from build123d import *

# Parameters (mm, degrees)
BOSS_EXTRUDE3_DEPTH = 10
BOSS_EXTRUDE4_DEPTH = 20
SKETCH2_R           = 2
SKETCH2_R_2         = 3
CUT_EXTRUDE1_DEPTH  = 40
FILLET3_R           = 10
FILLET4_R           = 10
FILLET5_R           = 5
FILLET6_R           = 5
FILLET7_R           = 5
FILLET8_R           = 5


with BuildPart() as part:
    # Sketch1 → Boss-Extrude3 (new, symmetric)
    with BuildSketch(Plane.XY):
        with BuildLine():
            Line((-6.014924663, 62.244051207), (6.208553437, 44.207596014))
            ThreePointArc((6.208553437, 44.207596014), (7.257156315, 41.893061598), (7.472748917, 39.361232736))
            Line((7.472748917, 39.361232736), (2.362176037, -20.425844843))
            ThreePointArc((2.362176037, -20.425844843), (7.015315923, -46.134373754), (24, -65.986342835))
            Line((24, -65.986342835), (31.161941742, -80.882336991))
            ThreePointArc((31.161941742, -80.882336991), (1.523988114, -56.838882139), (-7.619240262, -19.78625212))
            Line((-7.619240262, -19.78625212), (-7.50208553, 38.961677125))
            Line((-7.50208553, 38.961677125), (-13.173612773, 58.905900119))
            ThreePointArc((-13.173612773, 58.905900119), (-11.01662621, 63.625231148), (-6.014924663, 62.244051207))
        make_face()
        with BuildLine():
            Line((-7.499985087, 40.014956421), (-7.500014913, 40))
            ThreePointArc((-7.500014913, 40), (-7.499996272, 40.007478214), (-7.499985087, 40.014956421))
        make_face(mode=Mode.SUBTRACT)
    extrude(amount=BOSS_EXTRUDE3_DEPTH, both=True)

    # Sketch1<4> → Boss-Extrude4 (add, symmetric)
    with BuildSketch(Plane.XY):
        with BuildLine():
            ThreePointArc((25.760539384, -46.570125255), (39.455220381, -67.725242398), (47.426258953, -91.632266743))
            Line((47.426258953, -91.632266743), (38.413830656, -95.965410657))
            Line((38.413830656, -95.965410657), (31.161941742, -80.882336991))
            Line((31.161941742, -80.882336991), (24, -65.986342835))
            Line((24, -65.986342835), (16.748111086, -50.903269169))
            Line((16.748111086, -50.903269169), (25.760539384, -46.570125255))
        make_face()
    extrude(amount=BOSS_EXTRUDE4_DEPTH, both=True)

    # Sketch2 → Cut-Extrude1 (cut)
    with BuildSketch(Plane.XY.offset(10)):
        with Locations((-9.326153163, 60)):
            Circle(SKETCH2_R)
        with Locations((0, 40)):
            Circle(SKETCH2_R_2)
    extrude(amount=-CUT_EXTRUDE1_DEPTH, mode=Mode.SUBTRACT)

    # Fillet3
    fillet3_edges = [part.edges().sort_by_distance(p)[0] for p in [
        (-7.50208553, 38.961677125, 0),
    ]]
    fillet(fillet3_edges, radius=FILLET3_R)

    # Fillet4
    # the kernel refuses this fillet: 10 mm, written as the material it adds along each edge
    with BuildSketch(Plane(origin=(-7.619240262, -19.78625212, -10), x_dir=(0.0019941894265581785, 0.9999980116022886, 0), z_dir=(0, 0, 1))) as fillet4_piece_1:
        with BuildLine():
            CenterArc((0.38347882, 10), FILLET4_R, 265.770794781, 4.229205219)
            ThreePointArc((-0.353986639, 0.027229838), (-0.176973179, 0.013876746), (0, 0))
            Line((0, 0), (0.38347882, 0))
        make_face()
    extrude(amount=20)

    # Fillet5
    fillet5_edges = [part.edges().sort_by_distance(p)[0] for p in [
        (25.760539384, -46.570125255, 0),
    ]]
    fillet(fillet5_edges, radius=FILLET5_R)

    # Fillet6
    fillet6_edges = [part.edges().sort_by_distance(p)[0] for p in [
        (47.426258953, -91.632266743, 0),
    ]]
    fillet(fillet6_edges, radius=FILLET6_R)

    # Fillet7
    fillet7_edges = [part.edges().sort_by_distance(p)[0] for p in [
        (16.748111086, -50.903269169, 0),
    ]]
    fillet(fillet7_edges, radius=FILLET7_R)

    # Fillet8
    fillet8_edges = [part.edges().sort_by_distance(p)[0] for p in [
        (38.413830656, -95.965410657, 0),
    ]]
    fillet(fillet8_edges, radius=FILLET8_R)


solid = part.part
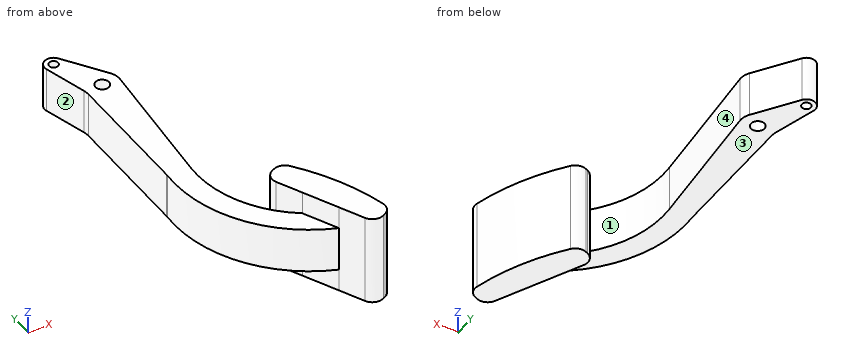
The listing builds one solid part. Answer for the finished solid, in the listing's coordinates (mm). Face numbers are marked on the shaded views. Give positions to 0.01 mm unless a question says otherwise; leave off trailing zeros. Write each loop counter-clockwise with the first axis right and the second up, starting at its lowest first coordinate (ties: lowest second). Pieces come first, ordered by that corner, then holes.
1) Section A-A (x = 0) is taken. Write down the section's boundary in (y, z).
2) For a pull along Y with two mould halves and no side action, classify the marked faces 1, 2, 3 and 4 as pulls with the +Y half, pulls with the -Y half, needs draft (parallel to the pull), parting line crosses it, or undercut.
3) Given P1, Ø6, axis at x = -5.5, z = 9, coming from the +Y side; P2, Ø6, axis at x = 18.5, z = 15.5, coming from the +Y side; P3, Ø22, axis at x = -1.5, y = -36.5, coming from the -Z side; P4, Ø5.5, axis at x = 0, y = 40, coming from the -Z side, each flat-ended and moving along its own axis, determine where each tip first touches the part or whether it passes through.
4) Find the intervals of material crossed by L1, parallel to Y at x = 0, z = 0; L2, parallel to Y at x = -2.5, z = 4; L3, parallel to X at y = -51.5, z = 1.5, in increasing order.
5) Section D-D (y = -78) is taken. Write down the section's boundary in (x, z), and give its area (3 significant figures).
6) Section C-C (z = 16.5) is taken. Write down the section's boundary in (x, y), and give its area (3 significant figures).
Response:
1. outline: (-54.3, -10) - (37, -10) - (37, 10) - (-54.3, 10) - close; (43, -10) - (53.37, -10) - (53.37, 10) - (43, 10) - close
2. face 1: undercut
2. face 2: pulls with the -Y half
2. face 3: needs draft
2. face 4: undercut
3. P1: stops at y = 63.91
3. P2: stops at y = -48.62
3. P3: stops at z = -10
3. P4: passes through
4. L1: y = -54.3 to 37, 43 to 53.37
4. L2: y = -49.38 to 38.34, 41.66 to 57.06
4. L3: x = -1.49 to 9.98, 18.73 to 29.66
5. outline: (24.66, -10) - (29.78, -10) - (29.78, -20) - (43.71, -20) - (43.71, 20) - (29.78, 20) - (29.78, 10) - (24.66, 10) - close
5. area: 660 mm2
6. outline: (18.91, -55.41) - (36.25, -91.46) arc R5 ccw to (42.92, -93.8) - (43.86, -93.35) arc R5 ccw to (46.56, -87.67) arc R100 ccw to (28.31, -49.72) arc R5 ccw to (22.2, -48.28) - (21.25, -48.74) arc R5 ccw to start
6. area: 589 mm2
